Geometry check sheet. Reference: the model listing, model coordinates, mm. A direction names the side the tool comes from. Round coordinates to 2 decimals unless told otherwise and drop trailing zeros. Use a Markdown table: item, result.
```python
from build123d import *

# Parameters (mm, degrees)
SKETCH1_R           = 2.15
BOSS_EXTRUDE1_DEPTH = 304.8
FILLET1_R           = 0.5


with BuildPart() as part:
    # Sketch1 → Boss-Extrude1 (new body)
    with BuildSketch(Plane.XY):
        Polygon((-10, 2.5), (-8.5, 2.5), (-8.5, 7.439339828), (-4, 2.939339828), (-4, 0), (-4, -2.939339828), (-8.5, -7.439339828), (-8.5, -2.5), (-10, -2.5), (-10, -10), (-2.5, -10), (-2.5, -8.5), (-7.439339828, -8.5), (-2.939339828, -4), (0, -4), (2.939339828, -4), (7.439339828, -8.5), (2.5, -8.5), (2.5, -10), (10, -10), (10, -2.5), (8.5, -2.5), (8.5, -7.439339828), (4, -2.939339828), (4, 0), (4, 2.939339828), (8.5, 7.439339828), (8.5, 2.5), (10, 2.5), (10, 10), (2.5, 10), (2.5, 8.5), (7.439339828, 8.5), (2.939339828, 4), (0, 4), (-2.939339828, 4), (-7.439339828, 8.5), (-2.5, 8.5), (-2.5, 10), (-10, 10), align=None)
        with Locations(Location((0, 0, 0), (0, 0, 180))):
            Circle(SKETCH1_R, mode=Mode.SUBTRACT)
    extrude(amount=BOSS_EXTRUDE1_DEPTH)

    # Fillet1
    fillet1_edges = [part.edges().sort_by_distance(p)[0] for p in [
        (7.439339828, 8.5, 152.4),
        (2.5, 8.5, 152.4),
        (2.5, 10, 152.4),
        (10, 10, 152.4),
        (10, 2.5, 152.4),
        (8.5, 2.5, 152.4),
        (8.5, 7.439339828, 152.4),
        (8.5, -7.439339828, 152.4),
        (8.5, -2.5, 152.4),
        (10, -2.5, 152.4),
        (10, -10, 152.4),
        (2.5, -10, 152.4),
        (2.5, -8.5, 152.4),
        (7.439339828, -8.5, 152.4),
        (-7.439339828, -8.5, 152.4),
        (-2.5, -8.5, 152.4),
        (-2.5, -10, 152.4),
        (-10, -10, 152.4),
        (-10, -2.5, 152.4),
        (-8.5, -2.5, 152.4),
        (-8.5, -7.439339828, 152.4),
        (-8.5, 7.439339828, 152.4),
        (-8.5, 2.5, 152.4),
        (-10, 2.5, 152.4),
        (-10, 10, 152.4),
        (-2.5, 10, 152.4),
        (-2.5, 8.5, 152.4),
        (-7.439339828, 8.5, 152.4),
    ]]
    fillet(fillet1_edges, radius=FILLET1_R)


solid = part.part
```
Item 1: Material ranges on line 1 along Y through (x, z) = (0.5, 44.5); line 2 along Y through (x, z) = (-8, 239); line 3 along X through (y, z) = (0.25, 259), recorded low to high. Write a range as from..to.
Outcome:
| item | result |
|---|---|
| line 1 | y = -4..-2.09, 2.09..4 |
| line 2 | y = -10..-6.73, 6.73..10 |
| line 3 | x = -4..-2.14, 2.14..4 |
Item 2: Access from +Z, -Z, +X, -X, +Y, -Y to the whole of each face (thin tool, end or side, straight path). Record for faces 1 (the face through (-4, 0, 150)), 2 (the face through (6, -10, 150)).
Outcome:
| item | result |
|---|---|
| face 1 | +Z, -Z |
| face 2 | +Z, -Z, +X, -X, -Y |
Item 3: Go/stop test with flat-tipped pins: pin 1 (1 mm diameter, centred on y = 1, z = 158.5, fed in from +X); pin 2 (1.8 mm diameter, centred on x = -0.5, z = 117.5, fed in from +Y); pin 3 (1.8 mm diameter, centred on y = -1, z = 132, fed in from -X); pin 4 (6 mm diameter, centred on x = -0.5, y = 2, fed in from -Z). Record where each tip stops, or that it passes through.
Outcome:
| item | result |
|---|---|
| pin 1 | stops at x = 4 |
| pin 2 | stops at y = 4 |
| pin 3 | stops at x = -4 |
| pin 4 | stops at z = 0 |
Item 4: Mould release check, pull along X, two halves, no side actions. Record for faces 3 (the face through (0, 4, 150)), 4 (the face through (10, 6, 150)), 5 (the face through (-10, 6, 150)): +X half, -X half, draft (parallel to the pull), parting line (faces both ways), or undercut.
Outcome:
| item | result |
|---|---|
| face 3 | undercut |
| face 4 | +X half |
| face 5 | -X half |
